Can you work these out from the drawing? Everything is in mm from the part's minimum corner. Coordinates: 2 decimals unless noted, no trailing zeros. Order: outer loops, then holes, each group sorted by start corner. A loop starts at its lowest first (then second) coordinate and runs counter-clockwise, first axis right, second up. Notation, with made-up numbers: (-30, -32) - (-3, -32) arc R16 ccw to (-3, -26) - close; hole circle Ø1 at (66, -29.5). An arc over 180 degrees is marked (long way). Use a Markdown table: item, result. Add a question column.
(1) I want a section at C-C (z = 20). List the corners of the cut face in (x, y) for me.
(2) For pin 1 Ø1 at (x, y) = (25.5, 1.5) entering from +Z (1 decimal); pin 2 Ø1 at (y, z) = (0.5, 35) entering from -X (1 decimal), each with a flat end and sliding along its axis, tell me the tip position at first contact or that it passes through.
(3) If I drill on L1, parallel to Z at x = 20, y = 1.55; L2, parallel to Z at x = 15, y = 0.45 (1 decimal); L3, parallel to X at y = 0.9, z = 23.5, over which ranges is the centre line in solid material (lowest first)? Write a range as [from, to].
(4) I want a section at D-D (z = 13). List the corners of the cut face in (x, y) for me (1 decimal).
(5) I want a section at B-B (y = 1.55). List the corners of the cut face in (x, z) for me (1 decimal), and give its area (3 significant figures).
(6) I want a section at A-A (x = 20). List the corners of the cut face in (y, z) for me, and give its area (3 significant figures).
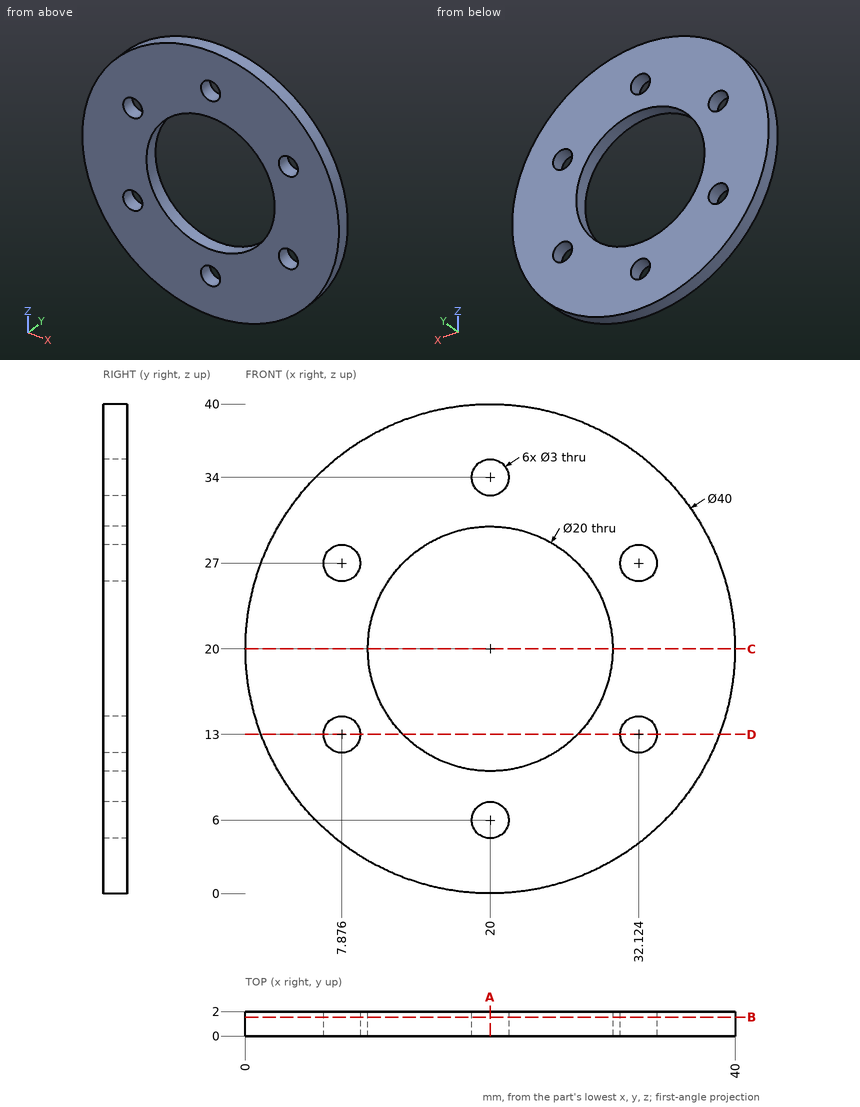
Answers follow:
| question | item | result |
|---|---|---|
| 1 | outline | (0, 0) - (10, 0) - (10, 2) - (0, 2) - close; (30, 0) - (40, 0) - (40, 2) - (30, 2) - close |
| 2 | pin 1 | stops at z = 39.4 |
| 2 | pin 2 | stops at x = 6.2 |
| 3 | L1 | z = [0, 4.5], [7.5, 10], [30, 32.5], [35.5, 40] |
| 3 | L2 | z = [0.6, 11.3], [28.7, 39.4] |
| 3 | L3 | x = [0.31, 10.63], [29.37, 39.69] |
| 4 | outline | (1.3, 0) - (6.4, 0) - (6.4, 2) - (1.3, 2) - close; (9.4, 0) - (12.9, 0) - (12.9, 2) - (9.4, 2) - close; (27.1, 0) - (30.6, 0) - (30.6, 2) - (27.1, 2) - close; (33.6, 0) - (38.7, 0) - (38.7, 2) - (33.6, 2) - close |
| 5 | outline | circle Ø40 at (20, 20); hole circle Ø3 at (7.9, 13); hole circle Ø3 at (7.9, 27); hole circle Ø20 at (20, 20); hole circle Ø3 at (20, 6); hole circle Ø3 at (20, 34); hole circle Ø3 at (32.1, 13); hole circle Ø3 at (32.1, 27) |
| 5 | area | 900 mm² |
| 6 | outline | (0, 0) - (2, 0) - (2, 4.5) - (0, 4.5) - close; (0, 7.5) - (2, 7.5) - (2, 10) - (0, 10) - close; (0, 30) - (2, 30) - (2, 32.5) - (0, 32.5) - close; (0, 35.5) - (2, 35.5) - (2, 40) - (0, 40) - close |
| 6 | area | 28.0 mm² |
